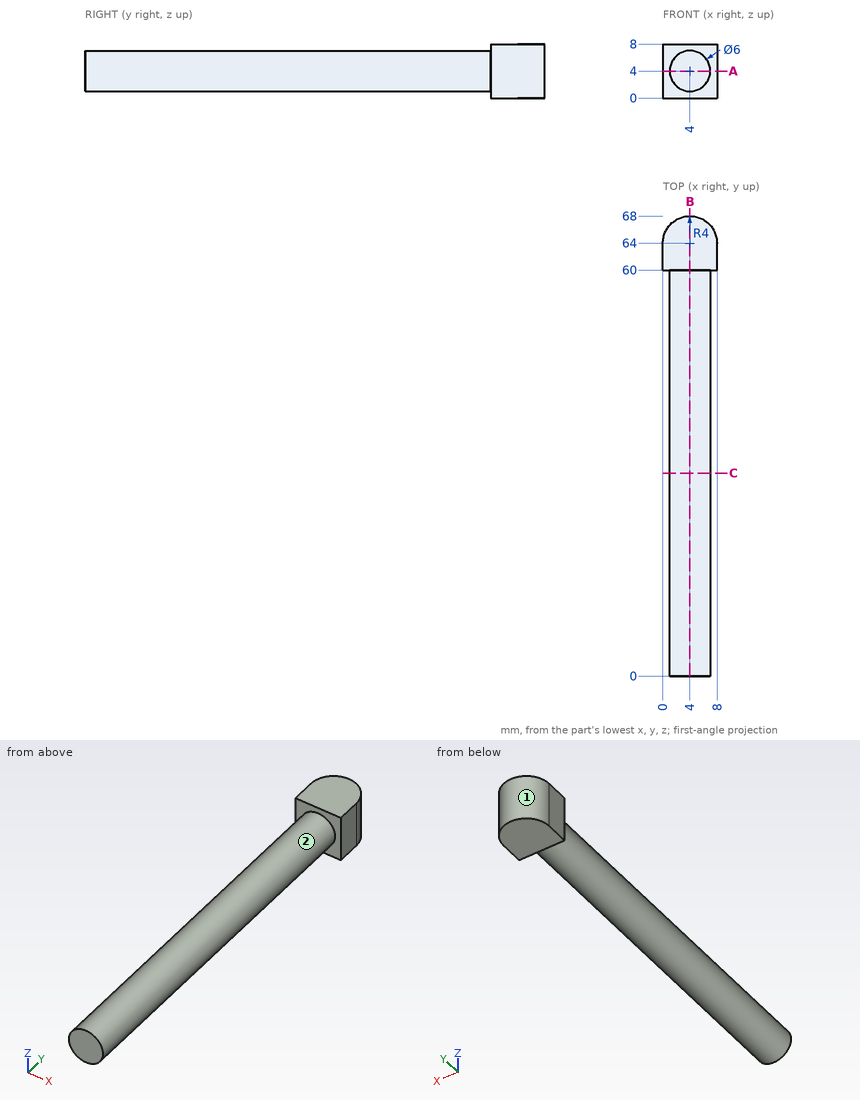
Verification items for this drawing (mm, ordinates from the low corner). A direction names the side the tool comes from. Give positions to 0.01 mm unless a question says otherwise; leave off trailing zeros. Loops run counter-clockwise (first coordinate to the right, second up) from the corner with the lowest first, then second, coordinate; pieces in that order, holes last.
(1) Set-up check for the marked faces 1 and 2: record each of +Z, -Z, +X, -X, +Y, -Y from which the full face is reachable in a straight line by a thin tool's end or side.
From the geometry:
face 1: +Z, -Z, +Y
face 2: -Y
(2) Section check A-A on z = 4. Record the cut outline in (x, y).
From the geometry:
outline: (0, 60) - (1, 60) - (1, 0) - (7, 0) - (7, 60) - (8, 60) - (8, 64) arc R4 ccw to (0, 64) - close
(3) Depth check by flat-ended pin: pin 1 Ø2 at (y, z) = (8, 4.5) entering from +X; pin 2 Ø3 at (x, y) = (3, 32) entering from +Z; pin 3 Ø1.5 at (y, z) = (20, 7) entering from -X. Enter the tip coordinate at first touch or a pass-through.
From the geometry:
pin 1: stops at x = 7
pin 2: stops at z = 7
pin 3: stops at x = 2.02
(4) Section check C-C on y = 30. Record the cut outline in (x, z), then the cut area to 3 significant figures.
From the geometry:
outline: circle Ø6 at (4, 4)
area: 28.3 mm2
(5) Thickness scan on L1, parallel to Z at x = 4, y = 21; L2, parallel to X at y = 19, z = 3.75; L3, parallel to Y at x = 7.25, z = 7.5. Record the ranges inside material, lowest first.
From the geometry:
L1: z = 1 to 7
L2: x = 1.01 to 6.99
L3: y = 60 to 66.33
(6) Section check B-B on x = 4. Record the cut outline in (y, z), then the cut area to 3 significant figures.
From the geometry:
outline: (0, 1) - (60, 1) - (60, 0) - (68, 0) - (68, 8) - (60, 8) - (60, 7) - (0, 7) - close
area: 424 mm2
